Answer from the drawing. Dimensions are ordinates in mm from the lowest x, y and z of the part. Round coordinates to 2 decimals unless told otherwise and drop trailing zeros. Loops run counter-clockwise (first coordinate to the right, second up) from the corner with the lowest first, then second, coordinate; pieces in that order, holes last. Notation, with made-up numbers: (89, -4) - (141, -4) arc R25 ccw to (141, 14) - close; hole circle Ø2 at (37.25, 40.5). An arc over 180 degrees is marked (long way). Write item = value, one per line. Start each with the question number.
1) Section D-D, the plane z = 16.25 is taken. Determine the outline of the cut face in (x, y), and give its area (3 significant figures).
2) Straight lines are drawn through the part: line 1 along Z through (x, y) = (3, 0.35); line 2 along Z through (x, y) = (2, 1.25); line 3 along Z through (x, y) = (10, 0.45). For each, find the intervals that lie inside material, in ascending order.
3) Section C-C, the plane y = 0.55 is taken. Determine the outline of the cut face in (x, z).
4) Section B-B, the plane z = 6 is taken. Determine the outline of the cut face in (x, y).
5) Given pin 1 Ø3.5 at (x, z) = (3, 3) entering from -Y; pin 2 Ø0.8 at (x, y) = (8, 0.5) entering from +Z, each flat-ended and moving along its own axis, determine where each tip first touches the part or whether it passes through.
6) Section A-A, the plane x = 3 is taken. Determine the outline of the cut face in (y, z).
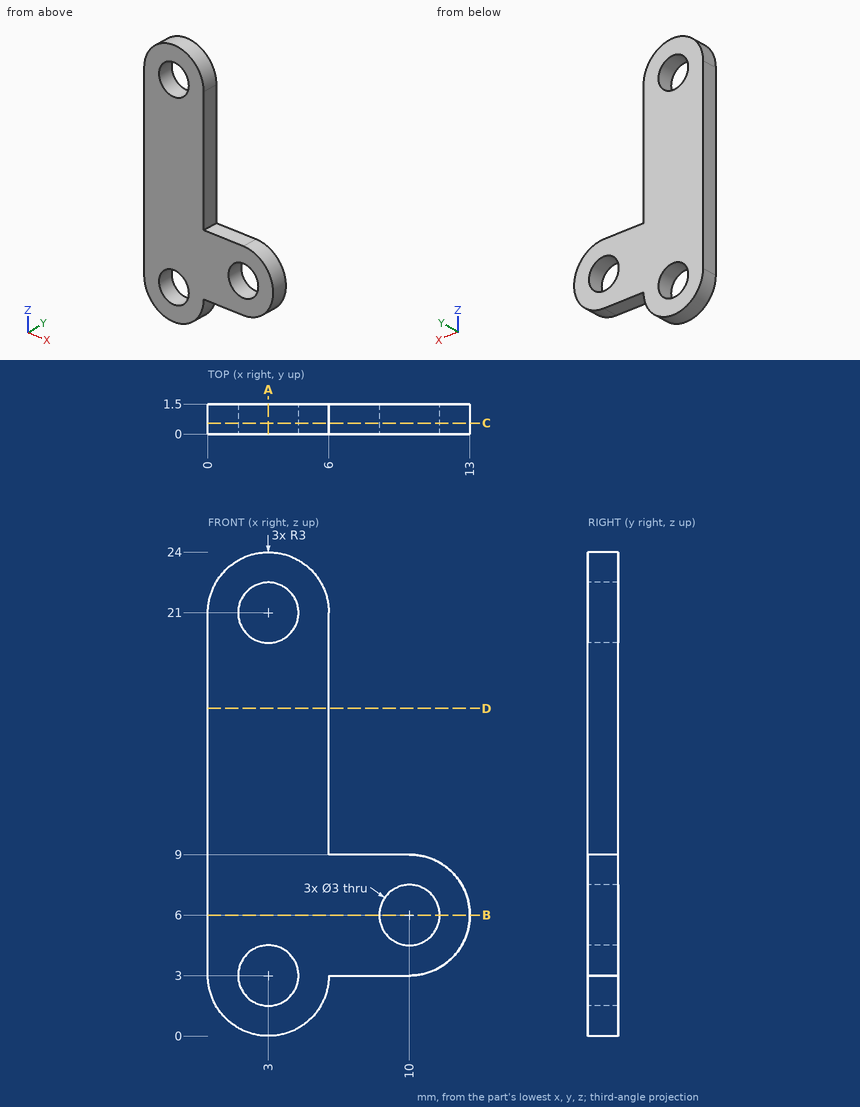
Geometry check:
q1.outline = (0, 0) - (6, 0) - (6, 1.5) - (0, 1.5) - close
q1.area = 9.00 mm2
q2.line_1 = 0 to 1.5, 4.5 to 19.5, 22.5 to 24
q2.line_2 = 0.17 to 1.88, 4.12 to 19.88, 22.12 to 23.83
q2.line_3 = 3 to 4.5, 7.5 to 9
q3.outline = (0, 3) arc R3 ccw to (6, 3) - (10, 3) arc R3 ccw to (10, 9) - (6, 9) - (6, 21) arc R3 ccw to (0, 21) - close; hole circle Ø3 at (3, 3); hole circle Ø3 at (3, 21); hole circle Ø3 at (10, 6)
q4.outline = (0, 0) - (8.5, 0) - (8.5, 1.5) - (0, 1.5) - close; (11.5, 0) - (13, 0) - (13, 1.5) - (11.5, 1.5) - close
q5.pin_1 = 0
q5.pin_2 = 9
q6.outline = (0, 0) - (1.5, 0) - (1.5, 1.5) - (0, 1.5) - close; (0, 4.5) - (1.5, 4.5) - (1.5, 19.5) - (0, 19.5) - close; (0, 22.5) - (1.5, 22.5) - (1.5, 24) - (0, 24) - close
